from build123d import *

# Parameters (mm, degrees)
F1_DEPTH = 2.54
F2_W     = 92.49156
F2_H     = 2.878541
F3_DEPTH = 25.4
F4_W     = 92.49156
F4_H     = 3.52044
F5_DEPTH = 25.4
F6_W     = 86.36
F6_H     = 3.499337
F7_DEPTH = 19.05


with BuildPart() as f1:
    # F0 (on Top) → F1 (new body)
    with BuildSketch(Plane.XY):
        with BuildLine():
            Line((-45.902735, 0), (45.902735, 0))
            ThreePointArc((45.902735, 0), (0, 45.902735), (-45.902735, 0))
        make_face()
    extrude(amount=F1_DEPTH)

    # F2 (on Top) → F3 (join)
    with BuildSketch(Plane.XY):
        with Locations((0.16002, 1.43927)):
            Rectangle(F2_W, F2_H)
    extrude(amount=F3_DEPTH)

    # F4 (on Top) → F5 (join)
    with BuildSketch(Plane.XY):
        with Locations((-0.37846, 4.958801)):
            Rectangle(F4_W, F4_H)
    extrude(amount=F5_DEPTH)

    # F6 (on Top) → F7 (cut)
    with BuildSketch(Plane.XY):
        with Locations((-0.358611, 1.749668)):
            Rectangle(F6_W, F6_H)
    extrude(amount=F7_DEPTH, mode=Mode.SUBTRACT)


solid = f1.part
Read the model definition and answer for the solid it produces. Units are mm, in the model's axes. A direction names the side the tool comes from. Give positions to 0.01 mm unless a question says otherwise; leave off trailing zeros. Write each loop counter-clockwise with the first axis right and the second up, starting at its lowest first coordinate (ties: lowest second). Pieces come first, ordered by that corner, then holes. Notation, with made-up numbers: M -29.75,45.25 L 9.25,45.25 A19 cw 9.25,80.25 Z; hole C 68,64 d5. An arc over 180 degrees is marked long. One line per item, written item: value. Start each with the question number.
(1) Determine the mould class of faces 1 (the flat face through (-43.539, 2, 9)), 2 (the cylindrical face through (0.915, 45.894, 1.252)), 3 (the flat face through (-1, 23, 0)) for opening direction X: pulls with the +X half, pulls with the -X half, needs draft (parallel to the pull), parting line crosses it, or undercut.
(2) Find section A-A (x = -13). Determine the outline of the cut face in (y, z).
(3) A tool of negligible diameter and unlimited length cuts with its end or side. For faces 4 (the flat face through (-46.086, 1, 13)), 5 (the flat face through (45.867, 5, 13)), 6 (the flat face through (-1, 22, 2.54)), 7 (the flat face through (-1, 3.499, 9)), from which of +Z, -Z, +X, -X, +Y, -Y can it reach the whole face along a straight path? Write none if from no direction.
(4) Find section B-B (z = 17.25). Determine the outline of the cut face in (x, y).
(5) Find the intervals of material crossed by line 1 (Y direction, x = -20, z = 6); line 2 (Z direction, x = -31.5, y = 19); line 3 (X direction, y = 19.5, z = 1.25), in increasing order.
(6) Find section D-D (y = 30). Determine the outline of the cut face in (x, z).
(7) Find section C-C (x = 18.5). Determine the outline of the cut face in (y, z).
(8) Flat-ended cylindrical pins translate along their axes: pin 1 Ø12 at (x, y) = (25, 32) entering from -Z; pin 2 Ø9.5 at (x, z) = (2.5, 11) entering from -Y; pin 3 Ø6 at (x, y) = (0, 15) entering from +Z; pin 4 Ø7.5 at (x, z) = (10.5, 12.5) entering from +Y. Find the tip coordinate at first contact, or state that the pin passes through.
Results below:
1. face 1: undercut
1. face 2: parting line crosses it
1. face 3: needs draft
2. outline: M 0,19.05 L 2.88,19.05 L 2.88,25.4 L 0,25.4 Z; M 3.2,19.05 L 3.5,19.05 L 3.5,0 L 44.02,0 L 44.02,2.54 L 6.72,2.54 L 6.72,25.4 L 3.2,25.4 Z
3. face 4: +Z, -Z, -X, -Y
3. face 5: +Z, -Z, +X, +Y
3. face 6: +Z, +X, -X, +Y
3. face 7: -Z, -Y
4. outline: M -46.62,3.2 L -43.54,3.2 L -43.54,3.5 L 42.82,3.5 L 42.82,3.2 L 45.87,3.2 L 45.87,6.72 L -46.62,6.72 Z; M -46.09,0 L -43.54,0 L -43.54,2.88 L -46.09,2.88 Z; M 42.82,0 L 46.41,0 L 46.41,2.88 L 42.82,2.88 Z
5. line 1: y = 3.5 to 6.72
5. line 2: z = 0 to 2.54
5. line 3: x = -41.55 to 41.55
6. outline: M -34.74,0 L 34.74,0 L 34.74,2.54 L -34.74,2.54 Z
7. outline: M 0,19.05 L 2.88,19.05 L 2.88,25.4 L 0,25.4 Z; M 3.2,19.05 L 3.5,19.05 L 3.5,0 L 42.01,0 L 42.01,2.54 L 6.72,2.54 L 6.72,25.4 L 3.2,25.4 Z
8. pin 1: stops at z = 0
8. pin 2: stops at y = 3.5
8. pin 3: stops at z = 2.54
8. pin 4: stops at y = 6.72
